CAD build for the part. Positions are in the model's coordinates, mm. Face numbers are marked on the shaded views. A direction names the side the tool comes from. Round coordinates to 2 decimals unless told otherwise and drop trailing zeros. Loops run counter-clockwise (first coordinate to the right, second up) from the corner with the lowest first, then second, coordinate; pieces in that order, holes last. Notation, with made-up numbers: M -7.5,87.5 L 46.5,87.5 A24 ccw 46.5,100.5 Z; hole C 44,2 d3. An arc over 180 degrees is marked long. Use a Markdown table: item, result. Add a question column.
(1) Band-saw the part on C-C, the plane x = 276. Write the cut outline in (y, z), and give its area (3 significant figures).
(2) Which spindle directions (+Z, -Z, +X, -X, +Y, -Y) get a long thin tool onto all of the face, cutting with end or side? Do the marked faces 1, 2, 3, 4 and 5. Say none if no direction does.
(3) Band-saw the part on A-A, the plane y = 0. Write the cut outline in (x, z) (3 decimals).
(4) Wall check: L1, parallel to X at y = 23.5, z = 11; L2, parallel to Z at x = 285, y = -7.5; L3, parallel to Z at x = 111, y = -12. Give the ranges that are in metal, low to high.
(5) Flat gauge pins, fed straight in: P1, Ø2, axis at y = 0.5, z = -21.5, coming from the +X side; P2, Ø3, axis at x = 89.5, z = 14, coming from the -Y side; P3, Ø2, axis at x = 98, y = -8, coming from the -Z side. Where does each tip first touch, or does it go through?
(6) Band-saw the part on D-D, the plane x = 130.5. Write the cut outline in (y, z).
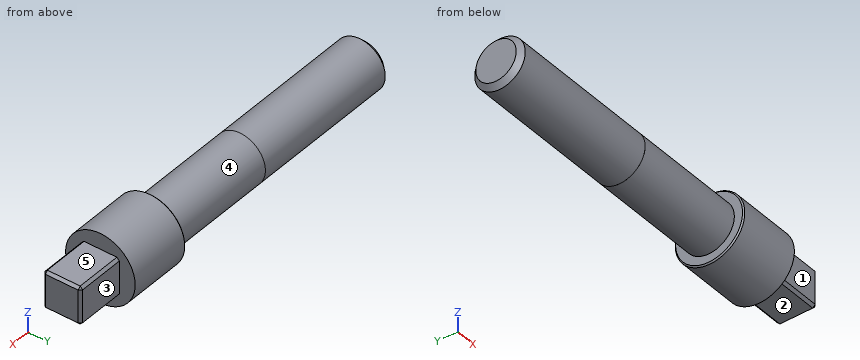
from build123d import *

# Parameters (mm, degrees)
SKETCH_1_R          = 20
EXTRUDE_1_DEPTH     = 215
SKETCH_2_R          = 27.5
EXTRUDE_2_DEPTH     = 51
SKETCH_3_W          = 30
SKETCH_3_H          = 30
EXTRUDE_3_DEPTH     = 39
CHAMFER_2_SIZE      = 1
CHAMFER_3_SIZE      = 2
SKETCH_4_R          = 20
SKETCH_4_R_2        = 19.975
CUT_EXTRUDE_1_DEPTH = 125
CHAMFER_4_SIZE      = 4


with BuildPart() as part:
    # 草图1 → 凸台-拉伸1 (new body)
    with BuildSketch(Plane(origin=(0, 0, 0), x_dir=(0, -1, 0), z_dir=(1, 0, 0))):
        with Locations(Location((0, 0, 0), (0, 0, 90))):
            Circle(SKETCH_1_R)
    extrude(amount=EXTRUDE_1_DEPTH)

    # 草图2 → 凸台-拉伸2 (add)
    with BuildSketch(Plane(origin=(215, 0, 0), x_dir=(0, -1, 0), z_dir=(1, 0, 0))):
        with Locations(Location((0, 0, 0), (0, 0, 180))):
            Circle(SKETCH_2_R)
    extrude(amount=EXTRUDE_2_DEPTH)

    # 草图3 → 凸台-拉伸3 (add)
    with BuildSketch(Plane(origin=(266, 0, 0), x_dir=(0, -1, 0), z_dir=(1, 0, 0))):
        Rectangle(SKETCH_3_W, SKETCH_3_H)
    extrude(amount=EXTRUDE_3_DEPTH)

    # 倒角2
    chamfer_2_edges = [part.edges().sort_by_distance(p)[0] for p in [
        (215, -27.5, 0),
    ]]
    chamfer(chamfer_2_edges, length=CHAMFER_2_SIZE)

    # 倒角3
    chamfer_3_edges = [part.edges().sort_by_distance(p)[0] for p in [
        (285.5, 15, -15),
        (285.5, 15, 15),
        (285.5, -15, 15),
        (285.5, -15, -15),
        (305, 15, 0),
        (305, 0, 15),
        (305, -15, 0),
        (305, 0, -15),
    ]]
    chamfer(chamfer_3_edges, length=CHAMFER_3_SIZE)

    # 草图4 → 切除-拉伸1 (cut)
    with BuildSketch(Plane(origin=(0, 0, 0), x_dir=(0, -1, 0), z_dir=(-1, 0, 0))):
        Circle(SKETCH_4_R)
        Circle(SKETCH_4_R_2, mode=Mode.SUBTRACT)
    extrude(amount=-CUT_EXTRUDE_1_DEPTH, mode=Mode.SUBTRACT)

    # 倒角4
    chamfer_4_edges = [part.edges().sort_by_distance(p)[0] for p in [
        (0, 19.975, 0),
    ]]
    chamfer(chamfer_4_edges, length=CHAMFER_4_SIZE)


solid = part.part
Return value:
| question | item | result |
|---|---|---|
| 1 | outline | M -15,-13 L -13,-15 L 13,-15 L 15,-13 L 15,13 L 13,15 L -13,15 L -15,13 Z |
| 1 | area | 892 mm^2 |
| 2 | face 1 | +Z, -Z, +X, -Y |
| 2 | face 2 | -Z, +X, +Y, -Y |
| 2 | face 3 | +Z, -Z, +X, +Y |
| 2 | face 4 | -X |
| 2 | face 5 | +Z, +X, +Y, -Y |
| 3 | outline | M 0,-15.975 L 4,-19.975 L 125,-19.975 L 125,-20 L 215,-20 L 215,-26.5 L 216,-27.5 L 266,-27.5 L 266,-15 L 303,-15 L 305,-13 L 305,13 L 303,15 L 266,15 L 266,27.5 L 216,27.5 L 215,26.5 L 215,20 L 125,20 L 125,19.975 L 4,19.975 L 0,15.975 Z |
| 4 | L1 | 215 to 266 |
| 4 | L2 | -15 to 15 |
| 4 | L3 | -15.97 to 15.97 |
| 5 | P1 | x = 266 |
| 5 | P2 | y = -15.58 |
| 5 | P3 | z = -18.71 |
| 6 | outline | C 0,0 d40 |
